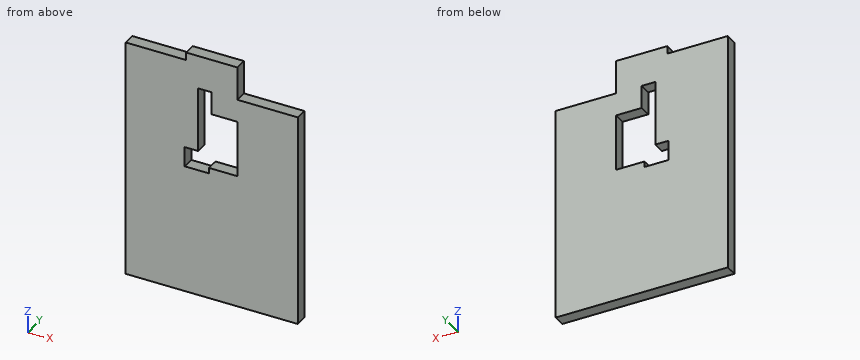
```python
from build123d import *

# Parameters (mm, degrees)
F0_W     = 181.5531998873
F0_H     = 102.3213416338
F0_W_2   = 127.5060996413
F0_H_2   = 48.1534004211
F0_H_3   = 54.1679412127
F0_W_3   = 54.047100246
F1_DEPTH = 25.4
F2_DEPTH = 25.4


with BuildPart() as f1:
    # F0 (on Front) → F1 (new body)
    with BuildSketch(Plane.XZ):
        with Locations((0, -139.9423852563)):
            Rectangle(F0_W, F0_H)
        Polygon((90.7765999436, -191.1030560732), (-90.7765999436, -191.1030560732), (-90.7765999436, -314.4985437393), (272.3297998309, -314.4985437393), (272.3297998309, -88.7817144394), (90.7765999436, -88.7817144394), align=None)
        Polygon((-90.7765999436, 88.7817144394), (-90.7765999436, -88.7817144394), (90.7765999436, -88.7817144394), (90.7765999436, -30.0107300282), (84.9582105875, -30.0107300282), (84.9582105875, -41.9930517673), (33.7925106287, -41.9930517673), (33.7925106287, 0), (36.7294996977, 0), (36.7294996977, 88.7817144394), align=None)
        Polygon((90.7765999436, -30.0107300282), (90.7765999436, -88.7817144394), (272.3297998309, -88.7817144394), (272.3297998309, 88.7817144394), (144.8237001896, 88.7817144394), (144.8237001896, 0), (144.8237001896, -30.0107300282), align=None)
        with Locations((-27.023550123, 112.85841465)):
            Rectangle(F0_W_2, F0_H_2)
        with Locations((-27.023550123, 164.0190854669)):
            Rectangle(F0_W_2, F0_H_3)
        with Locations((208.5767500103, 112.85841465)):
            Rectangle(F0_W_2, F0_H_2)
        with Locations((63.7530498207, 164.0190854669)):
            Rectangle(F0_W_3, F0_H_3)
        Polygon((90.7765999436, 118.6627522111), (90.7765999436, 88.7817144394), (144.8237001896, 88.7817144394), (144.8237001896, 136.9351148605), (90.7765999436, 136.9351148605), align=None)
        Polygon((36.7294996977, 207.5741589069), (36.7294996977, 191.1030560732), (90.7765999436, 191.1030560732), (90.7765999436, 136.9351148605), (144.8237001896, 136.9351148605), (144.8237001896, 207.5741589069), align=None)
    extrude(amount=-F1_DEPTH)

    # F2 (add): a face of the model
    f2_faces = [f1.faces().sort_by_distance(p)[0] for p in [
        (36.7294996977, 12.7, 68.4675574303),
    ]]
    extrude(f2_faces, amount=F2_DEPTH)


solid = f1.part
```
CAD build for the part. Positions are in the model's coordinates, mm. Round coordinates to 2 decimals unless told otherwise and drop trailing zeros. Write each loop counter-clockwise with the first axis right and the second up, starting at its lowest first coordinate (ties: lowest second). Pieces come first, ordered by that corner, then holes. Notation, with made-up numbers: (25, 49) - (72, 49) arc R23 cw to (72, 77) - close; hole circle Ø5 at (72, -38.5). An arc over 180 degrees is marked (long way). Return JSON: item names as keys, results as strings. Group by question number.
Item 1: Band-saw the part on B-B on y = 16. List the corners of the cut face in (x, z), plus the area to 3 significant figures.
Item 2: Band-saw the part on C-C on z = 56. List the corners of the cut face in (x, y), plus the area to 3 significant figures.
Item 3: Band-saw the part on A-A on z = -13. List the corners of the cut face in (x, y), plus the area to 3 significant figures.
Item 4: Probe probe 1 along X at (y, z) = (13.5, -39); probe 2 along Z at (x, y) = (82, 7.75); probe 3 along X at (y, z) = (13, 78). List the from-to ranges inside material, lowest first.
Item 5: Band-saw the part on D-D on x = 236.5. List the corners of the cut face in (y, z), plus the area to 3 significant figures.
Item 6: Flat gauge pins, fed straight in: pin 1 Ø12.5 at (x, y) = (-41, 11.5) entering from +Z; pin 2 Ø12.5 at (x, y) = (202.5, 14) entering from +Z; pin 3 Ø13 at (y, z) = (16, 195.5) entering from -X. Where does each tip first touch, or does it go through?
Resolved:
{
 "1": {"outline": "(-90.78, -314.5) - (272.33, -314.5) - (272.33, 136.94) - (144.82, 136.94) - (144.82, 207.57) - (36.73, 207.57) - (36.73, 191.1) - (-90.78, 191.1) - close; hole (33.79, -41.99) - (84.96, -41.99) - (84.96, -30.01) - (144.82, -30.01) - (144.82, 88.78) - (90.78, 88.78) - (90.78, 136.94) - (62.13, 136.94) - (62.13, 0) - (33.79, 0) - close", "area": "166,000 mm²"},
 "2": {"outline": "(-90.78, 0) - (62.13, 0) - (62.13, 25.4) - (-90.78, 25.4) - close; (144.82, 0) - (272.33, 0) - (272.33, 25.4) - (144.82, 25.4) - close", "area": "7,120 mm²"},
 "3": {"outline": "(-90.78, 0) - (33.79, 0) - (33.79, 25.4) - (-90.78, 25.4) - close; (144.82, 0) - (272.33, 0) - (272.33, 25.4) - (144.82, 25.4) - close", "area": "6,400 mm²"},
 "4": {"probe 1": "x = -90.78 to 33.79, 84.96 to 272.33", "probe 2": "z = -314.5 to -41.99, 136.94 to 207.57", "probe 3": "x = -90.78 to 62.13, 144.82 to 272.33"},
 "5": {"outline": "(0, -314.5) - (25.4, -314.5) - (25.4, 136.94) - (0, 136.94) - close", "area": "11,500 mm²"},
 "6": {"pin 1": "stops at z = 191.1", "pin 2": "stops at z = 136.94", "pin 3": "stops at x = -90.78"}
}
